Design review of the part built by this model. Coordinates are the model's own, in mm. A direction names the side the tool comes from. Coordinates: 2 decimals unless noted, no trailing zeros. Loops run counter-clockwise (first coordinate to the right, second up) from the corner with the lowest first, then second, coordinate; pieces in that order, holes last.
Q1. Add section B-B on z = 76.2. Give the boundary of the cut face in (x, y).
Q2. Machinability: for faces 1 (the face through (-3, 81, 6.35)), 2 (the face through (1.253, 33.626, 69.975)), 3 (the face through (-11.745, 2.421, 56.481)), which of the approach directions +Z, -Z, +X, -X, +Y, -Y give a long, thin tool a straight path to every point of the face, cutting with its end or side? Answer none if there is none.
Q3. For P1, Ø6, axis at x = 0, z = 0, coming from the +Y side; P2, Ø4, axis at x = 7, z = 32.5, coming from the -Y side; P3, Ø10, axis at x = 6, z = 0, coming from the +Y side (3 decimals), all flat-tipped, find the tip position at first contact; note any pin that passes through.
Q4. Wall thickness on probe 1 along Z at (x, y) = (0, 10); probe 2 along X at (y, z) = (10.75, 0); probe 3 along Z at (x, y) = (0, 4.25): over which ranges is each line inside the solid? List them lowest first.
Q5. Add section D-D on z = 63.5. Give the boundary of the cut face in (x, y) (3 decimals), and give its area (3 significant figures).
Q6. Add section A-A on x = -6.75. Give the boundary of the cut face in (y, z) (3 decimals), and give its area (3 significant figures).
Autodesk Inventor part; units mm, degrees
ref_plane "YZ Plane" through (0, 0, 0) normal (1, 0, 0) x (0, 1, 0)
ref_plane "XZ Plane" through (0, 0, 0) normal (0, 1, 0) x (-1, 0, 0)
ref_plane "XY Plane" through (0, 0, 0) normal (0, 0, 1) x (1, 0, 0)
sketch "Sketch1" plane through (0, 0, 0) normal (0, 1, 0) x (-1, 0, 0)
  circle A0 centre (0, 0) radius 2.2479
  line L0 (0, 0) -> (0, 76.2) construction
  circle A1 centre (0, 76.2) radius 2.2479
  line L1 (9.525, 82.55) -> (-9.525, 82.55)
  line L2 (-12.7, 79.375) -> (-12.7, -3.175)
  line L3 (-9.525, -6.35) -> (9.525, -6.35)
  line L4 (12.7, -3.175) -> (12.7, 79.375)
  line L5 (0, 0) -> (0, 55.5752) construction
  line L6 (12.7, 55.5752) -> (-12.7, 55.5752) construction
  line L7 (12.7, 55.5752) -> (-12.7, 55.5752)
  arc A2 (12.7, 79.375) -> (9.525, 82.55) centre (9.525, 79.375) ccw
  arc A3 (-9.525, 82.55) -> (-12.7, 79.375) centre (-9.525, 79.375) ccw
  arc A4 (9.525, -6.35) -> (12.7, -3.175) centre (9.525, -3.175) ccw
  arc A5 (-12.7, -3.175) -> (-9.525, -6.35) centre (-9.525, -3.175) ccw
  point P0 (-12.7, -6.35)
  point P1 (12.7, -6.35)
  dimension "d0" = 4.4958
  dimension "d1" = 4.4958
  dimension "d2" = 76.2
  dimension "d3" = 25.4
  dimension "d4" = 12.7
  dimension "d5" = 6.35
  dimension "d6" = 6.35
  dimension "d7" = 55.5752
  dimension "d8" = 3.175
extrude "Extrusion1" add sketch "Sketch1" along normal blind 53.975
sketch "Sketch2" plane through (0, 53.975, 0) normal (0, 1, 0) x (1, 0, 0)
  line L0 (12.7, -79.375) -> (12.7, 3.175)
  arc A0 (12.7, 3.175) -> (9.525, 6.35) centre (9.525, 3.175) ccw
  line L1 (9.525, 6.35) -> (-9.525, 6.35)
  arc A1 (-9.525, 6.35) -> (-12.7, 3.175) centre (-9.525, 3.175) ccw
  line L2 (-12.7, 3.175) -> (-12.7, -79.375)
  arc A2 (-12.7, -79.375) -> (-9.525, -82.55) centre (-9.525, -79.375) ccw
  line L3 (-9.525, -82.55) -> (9.525, -82.55)
  arc A3 (9.525, -82.55) -> (12.7, -79.375) centre (9.525, -79.375) ccw
  circle A4 centre (0, 0) radius 2.2479
  circle A5 centre (0, -76.2) radius 2.2479
  line L4 (5.5044, -82.55) -> (12.7, 0)
  line L5 (12.7, -79.375) -> (12.7, 3.175)
  line L6 (-12.7, 0) -> (12.7, 0) construction
  line L7 (2.2479, -76.2) -> (6.0579, -76.2) construction
  line L8 (5.5044, -82.55) -> (12.7, -82.55)
  line L9 (12.7, -82.55) -> (12.7, 0)
  point P0 (12.7, 0)
  dimension "d14" = 3.81
extrude "Extrusion3" cut sketch "Sketch2" against normal through all contours A3 L3 L4 L0
fillet "Fillet2" radius 3.175 1 edges at (5.5044, 26.9875, 82.55)
sketch "Sketch3" plane through (0, 53.975, 0) normal (0, 1, 0) x (1, 0, 0)
  point P0 (0, 0)
extrude "Extrusion4" cut sketch "Sketch1" along normal blind 4.7752 contours L4 A4 L3 A5 L2 L7
fillet "Fillet3" radius 3.175 2 edges at (7.8557, 2.3876, 55.5752) (-12.7, 2.3876, 55.5752)
sketch "Sketch5" plane through (0, 53.975, 0) normal (0, 1, 0) x (1, 0, 0)
  circle A0 centre (0, -76.2) radius 2.2479
  circle A1 centre (0, 0) radius 2.2479
  arc A2 (2.5941, -82.55) -> (5.7571, -79.6507) centre (2.5941, -79.375) ccw
  line L0 (5.7571, -79.6507) -> (12.7, 0)
  line L1 (12.7, 0) -> (12.7, 3.175)
  arc A3 (12.7, 3.175) -> (9.525, 6.35) centre (9.525, 3.175) ccw
  line L2 (9.525, 6.35) -> (-9.525, 6.35)
  arc A4 (-9.525, 6.35) -> (-12.7, 3.175) centre (-9.525, 3.175) ccw
  line L3 (-12.7, 3.175) -> (-12.7, -79.375)
  arc A5 (-12.7, -79.375) -> (-9.525, -82.55) centre (-9.525, -79.375) ccw
  line L4 (-9.525, -82.55) -> (2.5941, -82.55)
  circle A6 centre (0, 0) radius 6.35 construction
  line L5 (6.35, 0) -> (6.35, 6.35)
  line L6 (0, -6.35) -> (-12.7, -6.35)
  arc A7 (0, -6.35) -> (6.35, 0) centre (0, 0) ccw
  line L7 (6.35, 6.35) -> (-12.7, 6.35)
  line L8 (-12.7, 6.35) -> (-12.7, -6.35)
  circle A8 centre (0, -76.2) radius 6.35 construction
  line L9 (0, -69.85) -> (-12.7, -69.85)
  line L10 (6.1837, -74.7564) -> (5.5044, -82.55)
  line L11 (5.5044, -82.55) -> (-12.7, -82.55)
  line L12 (-12.7, -82.55) -> (-12.7, -69.85)
  line L13 (-9.525, -82.55) -> (2.5941, -82.55)
  arc A9 (6.1837, -74.7564) -> (0, -69.85) centre (0, -76.2) ccw
  dimension "d21" = 12.7
  dimension "d22" = 12.7
extrude "Extrusion5" cut sketch "Sketch5" against normal blind 41.275 contours L4 A5 L3 L9 A9 L0 A2 | L3 A4 L2 L5 A7 L6
fillet "Fillet4" radius 3.175 1 edges at (6.1837, 33.3375, 74.7564)
fillet "Fillet5" radius 3.175 3 edges at (-12.7, 33.3375, 69.85) (-12.7, 33.3375, 6.35) (6.35, 33.3375, -6.35)
sketch "Sketch6" plane through (0, 53.975, 0) normal (0, 1, 0) x (1, 0, 0)
  arc A0 (12.7, 3.175) -> (6.35, 3.175) centre (9.525, 3.175) ccw
  line L0 (6.35, 3.175) -> (6.35, 0)
  arc A1 (0, -6.35) -> (6.35, 0) centre (0, 0) ccw
  line L1 (0, -6.35) -> (-9.525, -6.35)
  arc A2 (-9.525, -6.35) -> (-12.7, -9.525) centre (-9.525, -9.525) ccw
  line L2 (-12.7, -9.525) -> (-12.7, -66.675)
  arc A3 (-12.7, -66.675) -> (-9.525, -69.85) centre (-9.525, -66.675) ccw
  line L3 (-9.525, -69.85) -> (0, -69.85)
  arc A4 (2.4254, -70.3315) -> (0, -69.85) centre (0, -76.2) ccw
  arc A5 (2.4254, -70.3315) -> (6.8012, -67.6729) centre (3.6382, -67.3972) ccw
  line L4 (6.8012, -67.6729) -> (12.7, 0)
  line L5 (12.7, 0) -> (12.7, 3.175)
  point P0 (0, 0)
extrude "Extrusion6" add sketch "Sketch6" along normal blind 69.85
sketch "Sketch7" plane through (0, 123.825, 0) normal (0, 1, 0) x (1, 0, 0)
  line L0 (6.8012, -67.6729) -> (12.7, 0)
  line L1 (12.7, 0) -> (12.7, 3.175)
  arc A0 (12.7, 3.175) -> (6.35, 3.175) centre (9.525, 3.175) ccw
  line L2 (6.35, 3.175) -> (6.35, 0)
  arc A1 (0, -6.35) -> (6.35, 0) centre (0, 0) ccw
  line L3 (0, -6.35) -> (-9.525, -6.35)
  arc A2 (-9.525, -6.35) -> (-12.7, -9.525) centre (-9.525, -9.525) ccw
  line L4 (-12.7, -9.525) -> (-12.7, -66.675)
  arc A3 (-12.7, -66.675) -> (-9.525, -69.85) centre (-9.525, -66.675) ccw
  line L5 (-9.525, -69.85) -> (0, -69.85)
  arc A4 (2.4254, -70.3315) -> (0, -69.85) centre (0, -76.2) ccw
  arc A5 (2.4254, -70.3315) -> (6.8012, -67.6729) centre (3.6382, -67.3972) ccw
  line L6 (6.35, 0) -> (6.35, 3.175)
  arc A6 (9.525, 6.35) -> (6.35, 3.175) centre (9.525, 3.175) ccw
  line L7 (12.7, 0) -> (12.7, 3.175)
  arc A7 (12.7, 3.175) -> (6.35, 3.175) centre (9.525, 3.175) ccw
  line L8 (0, -6.35) -> (12.1465, -6.35)
  arc A8 (0, -6.35) -> (6.35, 0) centre (0, 0) ccw
  line L9 (12.1465, -6.35) -> (12.7, 0)
  arc A9 (0, -6.35) -> (6.35, 0) centre (0, 0) ccw
  point P0 (0, 0)
extrude "Extrusion8" cut sketch "Sketch7" against normal blind 57.15 contours L8 A1 L2 A0 L1 L0
fillet "Fillet6" radius 3.175 1 edges at (12.1465, 95.25, 6.35)
properties part number "INtk_016_PelletDeflector1" material "PC/ABS Plastic"
Entries:
1. outline: (-12.7, 0) - (-2.25, 0) - (-2.25, 12.7) - (-12.7, 12.7) - close; (2.25, 0) - (6.06, 0) - (6.06, 12.7) - (2.25, 12.7) - close
2. face 1: -Z, -X, +Y
2. face 2: +Z, -X, +Y
2. face 3: -Z, -X, -Y
3. P1: stops at y = 12.7
3. P2: stops at y = 4.78
3. P3: stops at y = 66.675
4. probe 1: z = -6.35 to -2.25, 2.25 to 73.95, 78.45 to 82.55
4. probe 2: x = -12.7 to -2.25, 2.25 to 12.7
4. probe 3: z = 55.58 to 73.95, 78.45 to 82.55
5. outline: (-12.7, 0) - (7.165, 0) - (7.165, 123.825) - (-12.7, 123.825) - close
5. area: 2,460 mm2
6. outline: (0, 55.575) - (4.775, 55.575) - (4.775, -6.35) - (12.7, -6.35) - (12.7, 6.35) - (123.825, 6.35) - (123.825, 69.85) - (12.7, 69.85) - (12.7, 82.55) - (0, 82.55) - close
6. area: 7,890 mm2
